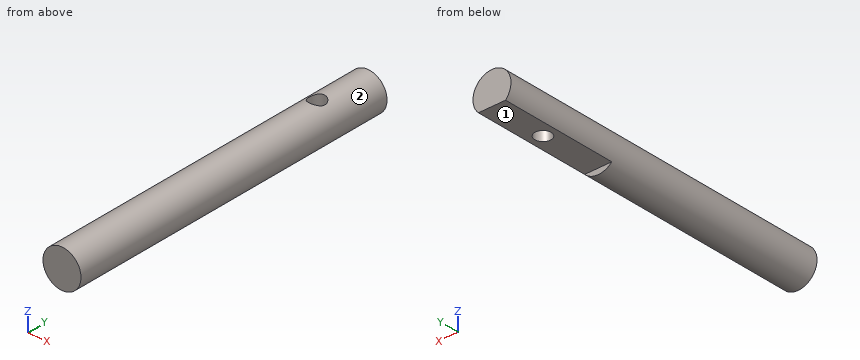
Autodesk Inventor part; units mm, degrees
ref_plane "YZ Plane" through (0, 0, 0) normal (1, 0, 0) x (0, 1, 0)
ref_plane "XZ Plane" through (0, 0, 0) normal (0, 1, 0) x (-1, 0, 0)
ref_plane "XY Plane" through (0, 0, 0) normal (0, 0, 1) x (1, 0, 0)
sketch "スケッチ2" plane through (0, 0, 0) normal (0, 1, 0) x (-1, 0, 0)
  circle A0 centre (0, 0) radius 4
  dimension "d0" = 8
extrude "押し出し1" add sketch "スケッチ2" along normal blind 72
sketch "スケッチ3" plane through (0, 72, 0) normal (0, 1, 0) x (1, 0, 0)
  line L0 (-4.1769, 6.014) -> (4.0611, 6.014)
  line L1 (4.0611, 6.014) -> (4.0611, 2.8)
  line L2 (4.0611, 2.8) -> (-4.1769, 2.8)
  line L3 (-4.1769, 2.8) -> (-4.1769, 6.014)
  point P0 (0, 0)
  dimension "d3" = 2.8
extrude "押し出し2" cut sketch "スケッチ3" against normal blind 25
sketch "スケッチ4" plane through (2.8566, 72, -2.8) normal (0, 0, -1) x (-1, 0, 0)
  line L0 (6.8566, 0) -> (-1.1434, 0)
  line L1 (2.8566, 0) -> (2.8566, -27.2038) construction
  circle A0 centre (2.8566, -12) radius 1.7
  point P0 (2.8566, -72)
  point P1 (5.7131, 0)
  point P2 (0, 0)
  dimension "d6" = 3.4
  dimension "d7" = 12
extrude "押し出し3" cut sketch "スケッチ4" against normal through all
properties part number "Rotary_Feedthorough_top"
Here's how the part is built. I have some questions about the finished solid (model axes, mm). Face numbers are marked on the shaded views. A direction names the side the tool comes from. Coordinates: 2 decimals unless noted, no trailing zeros. Order: outer loops, then holes, each group sorted by start corner. A loop starts at its lowest first (then second) coordinate and runs counter-clockwise, first axis right, second up. Notation, with made-up numbers: (-26.75, 63.25) -> (-17.75, 63.25) arc R29 cw to (-17.75, 97.25) -> close; hole circle Ø7 at (-14.75, 16.5). An arc over 180 degrees is marked (long way). Answer in a Markdown table with one row per item.
(1) I want a section at A-A on x = 0. List the corners of the cut face in (y, z) for me.
Answer key:
| item | result |
|---|---|
| outline | (0, -4) -> (47, -4) -> (47, -2.8) -> (58.3, -2.8) -> (58.3, 4) -> (0, 4) -> close; (61.7, -2.8) -> (72, -2.8) -> (72, 4) -> (61.7, 4) -> close |
(2) On a 3-axis mill with a long thin cutter (end or side, diameter ignored), from which of +Z, -Z, +X, -X, +Y, -Y can I reach the whole of each face in a straight line? I mean the marked faces 1 and 2. Say none if no direction works.
Answer key:
| item | result |
|---|---|
| face 1 | -Z, +X, -X, +Y |
| face 2 | +Y, -Y |
(3) Please list where these lines run through material, in increasing order: probe 1 along Y at (x, z) = (0, 1.5); probe 2 along Y at (x, z) = (0.5, -3.25); probe 3 along Y at (x, z) = (-1, 1.25).
Answer key:
| item | result |
|---|---|
| probe 1 | 0 to 58.3, 61.7 to 72 |
| probe 2 | 0 to 47 |
| probe 3 | 0 to 58.63, 61.37 to 72 |
(4) I want a section at C-C on y = 24.5. List the corners of the cut face in (x, z) for me, then the cut area to 3 significant figures.
Answer key:
| item | result |
|---|---|
| outline | circle Ø8 at (0, 0) |
| area | 50.3 mm^2 |
(5) Will these pins go through, and if not, where does the flat tip stop? pin 1 Ø1.7 at (x, y) = (0.5, 62) entering from -Z; pin 2 Ø1.5 at (x, y) = (1.5, 39.5) entering from +Z; pin 3 Ø1 at (y, z) = (41, -2.5) entering from +X; pin 4 Ø3 at (x, y) = (0, 60) entering from -Z.
Answer key:
| item | result |
|---|---|
| pin 1 | z = -2.8 |
| pin 2 | z = 3.93 |
| pin 3 | x = 3.46 |
| pin 4 | through |
(6) I want a section at D-D on y = 60. List the corners of the cut face in (x, z) for me, then the cut area to 3 significant figures.
Answer key:
| item | result |
|---|---|
| outline | (-2.86, -2.8) -> (-1.7, -2.8) -> (-1.7, 3.62) arc R4 ccw to start; (1.7, -2.8) -> (2.86, -2.8) arc R4 ccw to (1.7, 3.62) -> close |
| area | 22.8 mm^2 |
(7) I want a section at B-B on z = 0. List the corners of the cut face in (x, y) for me.
Answer key:
| item | result |
|---|---|
| outline | (-4, 0) -> (4, 0) -> (4, 72) -> (-4, 72) -> close; hole circle Ø3.4 at (0, 60) |
